Read the model definition and answer for the solid it produces. Units are mm, in the model's axes. A direction names the side the tool comes from. Coordinates: 2 decimals unless noted, no trailing zeros. Write each loop counter-clockwise with the first axis right and the second up, starting at its lowest first coordinate (ties: lowest second). Pieces come first, ordered by that corner, then holes. Notation, with made-up numbers: M 87.25,14.25 L 111.25,14.25 A30 cw 111.25,49.25 Z; hole C 41.5,40.5 d3. An arc over 180 degrees is marked long. Write item = value, one per line.
from build123d import *

# Parameters (mm, degrees)
F0_R     = 5
F0_R_2   = 2.5
F1_DEPTH = 10
F2_R     = 2.5
F3_DEPTH = 8
F4_START = -32
F4_DEPTH = 8
F5_DEPTH = 7


with BuildPart() as f1:
    # F0 (on Top) → F1 (new body)
    with BuildSketch(Plane.XY):
        with BuildLine():
            Line((26, 40), (-26, 40))
            ThreePointArc((-26, 40), (-31.6568542495, 37.6568542495), (-34, 32))
            Line((-34, 32), (-34, 8))
            ThreePointArc((-34, 8), (-31.6568542495, 2.3431457505), (-26, 0))
            Line((-26, 0), (26, 0))
            ThreePointArc((26, 0), (31.6568542495, 2.3431457505), (34, 8))
            Line((34, 8), (34, 32))
            ThreePointArc((34, 32), (31.6568542495, 37.6568542495), (26, 40))
        make_face()
        with Locations((-26, 8)):
            Circle(F0_R, mode=Mode.SUBTRACT)
        with Locations((26, 8)):
            Circle(F0_R, mode=Mode.SUBTRACT)
        with Locations((-26, 32)):
            Circle(F0_R, mode=Mode.SUBTRACT)
        with Locations((26, 32)):
            Circle(F0_R, mode=Mode.SUBTRACT)
        with Locations((-26, 32)):
            Circle(F0_R)
        with Locations((-26, 32)):
            Circle(F0_R_2, mode=Mode.SUBTRACT)
        with Locations((-26, 8)):
            Circle(F0_R)
        with Locations((-26, 8)):
            Circle(F0_R_2, mode=Mode.SUBTRACT)
        with Locations((26, 8)):
            Circle(F0_R)
        with Locations((26, 8)):
            Circle(F0_R_2, mode=Mode.SUBTRACT)
        with Locations((26, 32)):
            Circle(F0_R)
        with Locations((26, 32)):
            Circle(F0_R_2, mode=Mode.SUBTRACT)
        with Locations((26, 32)):
            Circle(F0_R_2)
        with Locations((26, 8)):
            Circle(F0_R_2)
        with Locations((-26, 8)):
            Circle(F0_R_2)
        with Locations((-26, 32)):
            Circle(F0_R_2)
    extrude(amount=F1_DEPTH)

    # F2 (on face) → F3 (join)
    with BuildSketch(Plane(origin=(0, 40, 0), x_dir=(-1, 0, 0), z_dir=(0, 1, 0))):
        with BuildLine():
            ThreePointArc((-14, 12.7841615349), (-14.9984986023, 10.9417491732), (-16.8705539605, 10))
            Line((-16.8705539605, 10), (16.922764346, 10))
            ThreePointArc((16.922764346, 10), (14.6793579532, 10.8135287538), (13.4788519072, 12.8759269962))
            Line((13.4788519072, 12.8759269962), (6.8878248776, 49.2481460075))
            ThreePointArc((6.8878248776, 49.2481460075), (6.9718998179, 48.6265883246), (7, 48))
            ThreePointArc((7, 48), (-0.673098164, 41.0324366625), (-6.8705539605, 49.3399583115))
            Line((-6.8705539605, 49.3399583115), (-14, 12.7841615349))
        make_face()
        with BuildLine():
            ThreePointArc((6.8878248776, 49.2481460075), (0.0467113041, 54.999844145), (-6.8705539605, 49.3399583115))
            ThreePointArc((-6.8705539605, 49.3399583115), (-0.673098164, 41.0324366625), (7, 48))
            ThreePointArc((7, 48), (6.9718998179, 48.6265883246), (6.8878248776, 49.2481460075))
        make_face()
        with Locations((0, 48)):
            Circle(F2_R, mode=Mode.SUBTRACT)
    extrude(amount=-F3_DEPTH)

    # F2 (on face) → F4 (join)
    with BuildSketch(Plane(origin=(0, 40, 0), x_dir=(-1, 0, 0), z_dir=(0, 1, 0)).offset(F4_START)):
        with BuildLine():
            ThreePointArc((-14, 12.7841615349), (-14.9984986023, 10.9417491732), (-16.8705539605, 10))
            Line((-16.8705539605, 10), (16.922764346, 10))
            ThreePointArc((16.922764346, 10), (14.6793579532, 10.8135287538), (13.4788519072, 12.8759269962))
            Line((13.4788519072, 12.8759269962), (6.8878248776, 49.2481460075))
            ThreePointArc((6.8878248776, 49.2481460075), (6.9718998179, 48.6265883246), (7, 48))
            ThreePointArc((7, 48), (-0.673098164, 41.0324366625), (-6.8705539605, 49.3399583115))
            Line((-6.8705539605, 49.3399583115), (-14, 12.7841615349))
        make_face()
        with BuildLine():
            ThreePointArc((6.8878248776, 49.2481460075), (0.0467113041, 54.999844145), (-6.8705539605, 49.3399583115))
            ThreePointArc((-6.8705539605, 49.3399583115), (-0.673098164, 41.0324366625), (7, 48))
            ThreePointArc((7, 48), (6.9718998179, 48.6265883246), (6.8878248776, 49.2481460075))
        make_face()
        with Locations((0, 48)):
            Circle(F2_R, mode=Mode.SUBTRACT)
    extrude(amount=-F4_DEPTH)

    # F0 (on Top) → F5 (cut)
    with BuildSketch(Plane.XY):
        with Locations((26, 8)):
            Circle(F0_R_2)
        with Locations((26, 32)):
            Circle(F0_R_2)
        with Locations((-26, 32)):
            Circle(F0_R_2)
        with Locations((-26, 8)):
            Circle(F0_R_2)
    extrude(amount=F5_DEPTH, mode=Mode.SUBTRACT)

    # F7 (on offset) → F8 (revolve, cut)
    with BuildSketch(Plane.XZ.offset(-8)):
        Polygon((-21, 10), (-26, 10), (-26, 7), (-23.5, 7), align=None)
    revolve(axis=Axis((-26, 8, 8.5), (0, 0, -1)), mode=Mode.SUBTRACT)

    # F9 (on offset) → F10 (revolve, cut)
    with BuildSketch(Plane.XZ.offset(-8)):
        Polygon((26, 7), (26, 10), (21, 10), (23.5, 7), align=None)
    revolve(axis=Axis((26, 8, 8.5), (0, 0, -1)), mode=Mode.SUBTRACT)

    # F12 (on offset) → F13 (revolve, cut)
    with BuildSketch(Plane(origin=(0, 32, 0), x_dir=(-1, 0, 0), z_dir=(0, 1, 0))):
        Polygon((-26, 7), (-26, 10), (-31, 10), (-28.5, 7), align=None)
    revolve(axis=Axis((26, 32, 8.5), (0, 0, -1)), mode=Mode.SUBTRACT)

    # F14 (on offset) → F15 (revolve, cut)
    with BuildSketch(Plane(origin=(0, 32, 0), x_dir=(-1, 0, 0), z_dir=(0, 1, 0))):
        Polygon((31, 10), (26, 10), (26, 7), (28.5, 7), align=None)
    revolve(axis=Axis((-26, 32, 8.5), (0, 0, -1)), mode=Mode.SUBTRACT)


solid = f1.part
Item 1: Find section A-A (x = 0). Determine the outline of the cut face in (y, z).
Worked answers:
outline = M 0,0 L 40,0 L 40,45.5 L 32,45.5 L 32,10 L 8,10 L 8,45.5 L 0,45.5 Z; M 0,50.5 L 8,50.5 L 8,55 L 0,55 Z; M 32,50.5 L 40,50.5 L 40,55 L 32,55 Z
Item 2: For a pull along X with two mould halves and no side action, classify faces 3 (the face through (0, 40, 21)), 4 (the face through (24.16, 33.69, 3.45)), 5 (the face through (14.98, 4.06, 10.96)) as released by +X, released by -X, zero draft, split by the parting line, or undercut.
Worked answers:
face_3 = zero draft
face_4 = undercut
face_5 = released by +X
Item 3: Which of the six approach directions +Z, -Z, +X, -X, +Y, -Y give full straight-line access (tool end or side, diameter ignored) to faces 1 (the face through (0, 8, 28)), 2 (the face through (0, 20, 0))?
Worked answers:
face_1 = +Z, +X, -X
face_2 = -Z, +X, -X, +Y, -Y
Item 4: Consider line 1 along Y through (x, z) = (26, 5.75); line 2 along Z through (x, y) = (0, 37); line 3 along Y through (x, z) = (-28, 6). Determine where each line is inside the solid, lowest interval first. Write a range as from..to.
Worked answers:
line_1 = 0..5.5, 10.5..29.5, 34.5..40
line_2 = 0..45.5, 50.5..55
line_3 = 0.25..6.5, 9.5..30.5, 33.5..39.75
Item 5: Flat-ended cylindrical pins translate along their axes: pin 1 (4 mm diameter, centred on x = -12, y = 29, fed in from +Z); pin 2 (1 mm diameter, centred on y = 35.5, z = 23, fed in from +X); pin 3 (6.5 mm diameter, centred on x = -26, y = 32, fed in from +Z). Find the tip coordinate at first contact, or state that the pin passes through.
Worked answers:
pin_1 = 10
pin_2 = 12.11
pin_3 = 7.9
Item 6: Find section B-B (z = 4.5). Determine the outline of the cut face in (x, y).
Worked answers:
outline = M -34,8 A8 ccw -26,0 L 26,0 A8 ccw 34,8 L 34,32 A8 ccw 26,40 L -26,40 A8 ccw -34,32 Z; hole C -26,8 d5; hole C -26,32 d5; hole C 26,8 d5; hole C 26,32 d5
Item 7: Find section D-D (x = 10). Determine the outline of the cut face in (y, z), and give its area (3 significant figures).
Worked answers:
outline = M 0,0 L 40,0 L 40,33.29 L 32,33.29 L 32,10 L 8,10 L 8,33.29 L 0,33.29 Z
area = 773 mm²
Item 8: Find section C-C (z = 21). Determine the outline of the cut face in (x, y), and give its area (3 significant figures).
Worked answers:
outline = M -12.01,0 L 12.4,0 L 12.4,8 L -12.01,8 Z; M -12.01,32 L 12.4,32 L 12.4,40 L -12.01,40 Z
area = 390 mm²
